from build123d import *

# Parameters (mm, degrees)
SKETCH_1_W                 = 50
SKETCH_1_H                 = 12
UPPER_CROSSBAR_DEPTH       = 28
SKETCH_2_R                 = 9.5
LOWER_GUIDE_SLEEVE_DEPTH   = 5
SKETCH_3_R                 = 6.2
SPINDLE_THROUGH_BORE_DEPTH = 60.774576536
UPPER_HINGE_EAR_DEPTH      = 6.7
SKETCH_6_R                 = 2.6
UPPER_HINGE_BORE_DEPTH     = 59.549124673
EXTRUDE_2_DEPTH            = 6.7
SKETCH_8_R                 = 2.6
CUT_EXTRUDE_2_DEPTH        = 59.549124673
OPPOSITE_HINGE_EAR_DEPTH   = 6.7
SKETCH_10_R                = 2.6
OPPOSITE_HINGE_BORE_DEPTH  = 59.549124673
EXTRUDE_4_DEPTH            = 6.7
SKETCH_12_R                = 2.6
CUT_EXTRUDE_4_DEPTH        = 59.549124673
SKETCH_14_W                = 20
SKETCH_14_H                = 2.2
ARM_SWING_CLEARANCE_DEPTH  = 7.2
SKETCH_15_W                = 20
SKETCH_15_H                = 2.2
CUT_EXTRUDE_6_DEPTH        = 7.2


with BuildPart() as part:
    # 草图1 → Upper_crossbar (new body)
    with BuildSketch(Plane.XY):
        with Locations((25, 6)):
            Rectangle(SKETCH_1_W, SKETCH_1_H)
    extrude(amount=UPPER_CROSSBAR_DEPTH)

    # 草图2 → Lower_guide_sleeve (add)
    with BuildSketch(Plane.XZ):
        with Locations(Location((25, 14, 0), (0, 0, 270))):
            Circle(SKETCH_2_R)
    extrude(amount=LOWER_GUIDE_SLEEVE_DEPTH)

    # 草图3 → Spindle_through_bore (cut, through all)
    with BuildSketch(Plane(origin=(0, 12, 0), x_dir=(1, 0, 0), z_dir=(0, 1, 0))):
        with Locations(Location((25, -14, 0), (0, 0, 270))):
            Circle(SKETCH_3_R)
    extrude(amount=-SPINDLE_THROUGH_BORE_DEPTH, mode=Mode.SUBTRACT)

    # 草图5 → Upper_hinge_ear (add)
    with BuildSketch(Plane.XY.offset(21.3)):
        Polygon((1, -10), (11, -10), (12, -7), (12, 1), (0, 1), (0, -7), align=None)
    extrude(amount=UPPER_HINGE_EAR_DEPTH)

    # 草图6 → Upper_hinge_bore (cut, through all)
    with BuildSketch(Plane.XY.offset(28)):
        with Locations((6, -5)):
            Circle(SKETCH_6_R)
    extrude(amount=-UPPER_HINGE_BORE_DEPTH, mode=Mode.SUBTRACT)

    # 草图7 → 凸台-拉伸2 (add)
    with BuildSketch(Plane.XY.offset(21.3)):
        Polygon((39, -10), (49, -10), (50, -7), (50, 1), (38, 1), (38, -7), align=None)
    extrude(amount=EXTRUDE_2_DEPTH)

    # 草图8 → 切除-拉伸2 (cut, through all)
    with BuildSketch(Plane.XY.offset(28)):
        with Locations((44, -5)):
            Circle(SKETCH_8_R)
    extrude(amount=-CUT_EXTRUDE_2_DEPTH, mode=Mode.SUBTRACT)

    # 草图9 → Opposite_hinge_ear (add)
    with BuildSketch(Plane.XY):
        Polygon((1, -10), (11, -10), (12, -7), (12, 1), (0, 1), (0, -7), align=None)
    extrude(amount=OPPOSITE_HINGE_EAR_DEPTH)

    # 草图10 → Opposite_hinge_bore (cut, through all)
    with BuildSketch(Plane(origin=(0, 0, 0), x_dir=(-1, 0, 0), z_dir=(0, 0, -1))):
        with Locations(Location((-6, -5, 0), (0, 0, 180))):
            Circle(SKETCH_10_R)
    extrude(amount=-OPPOSITE_HINGE_BORE_DEPTH, mode=Mode.SUBTRACT)

    # 草图11 → 凸台-拉伸4 (add)
    with BuildSketch(Plane.XY):
        Polygon((39, -10), (49, -10), (50, -7), (50, 1), (38, 1), (38, -7), align=None)
    extrude(amount=EXTRUDE_4_DEPTH)

    # 草图12 → 切除-拉伸4 (cut, through all)
    with BuildSketch(Plane(origin=(0, 0, 0), x_dir=(-1, 0, 0), z_dir=(0, 0, -1))):
        with Locations(Location((-44, -5, 0), (0, 0, 180))):
            Circle(SKETCH_12_R)
    extrude(amount=-CUT_EXTRUDE_4_DEPTH, mode=Mode.SUBTRACT)

    # 草图14 → Arm_swing_clearance (cut, symmetric)
    with BuildSketch(Plane.XY.offset(14)):
        with Locations((8, 0.9)):
            Rectangle(SKETCH_14_W, SKETCH_14_H)
    extrude(amount=ARM_SWING_CLEARANCE_DEPTH, both=True, mode=Mode.SUBTRACT)

    # 草图15 → 切除-拉伸6 (cut, symmetric)
    with BuildSketch(Plane.XY.offset(14)):
        with Locations((42, 0.9)):
            Rectangle(SKETCH_15_W, SKETCH_15_H)
    extrude(amount=CUT_EXTRUDE_6_DEPTH, both=True, mode=Mode.SUBTRACT)


solid = part.part
Verification items for the finished model (mm, model axes). A direction names the side the tool comes from. Coordinates: 2 decimals unless noted, no trailing zeros. Order: outer loops, then holes, each group sorted by start corner. A loop starts at its lowest first (then second) coordinate and runs counter-clockwise, first axis right, second up.
1. Sectioned sample at B-B, the plane y = -1. Record the cut outline in (x, z).
Results found:
outline: (0, 0) - (12, 0) - (12, 6.7) - (0, 6.7) - close; (0, 21.3) - (12, 21.3) - (12, 28) - (0, 28) - close; circle Ø19 at (25, 14); (38, 0) - (50, 0) - (50, 6.7) - (38, 6.7) - close; (38, 21.3) - (50, 21.3) - (50, 28) - (38, 28) - close; hole circle Ø12.4 at (25, 14)
2. Sectioned sample at C-C, the plane x = 25. Record the cut outline in (y, z).
Results found:
outline: (-5, 4.5) - (0, 4.5) - (0, 0) - (12, 0) - (12, 7.8) - (-5, 7.8) - close; (-5, 20.2) - (12, 20.2) - (12, 28) - (0, 28) - (0, 23.5) - (-5, 23.5) - close
3. Go/stop test with flat-tipped pins: pin 1 Ø1.5 at (y, z) = (-4, 10.5) entering from -X; pin 2 Ø1.5 at (x, z) = (10.5, 16.5) entering from -Y; pin 3 Ø2.5 at (y, z) = (0.5, 13) entering from +X. Record where each tip stops, or that it passes through.
Results found:
pin 1: stops at x = 15.91
pin 2: stops at y = 2
pin 3: stops at x = 34.5
4. Sectioned sample at D-D, the plane z = 24.5. Record the cut outline in (x, y), and give its area (3 significant figures).
Results found:
outline: (0, -7) - (1, -10) - (11, -10) - (12, -7) - (12, 0) - (38, 0) - (38, -7) - (39, -10) - (49, -10) - (50, -7) - (50, 12) - (0, 12) - close; hole circle Ø5.2 at (6, -5); hole circle Ø5.2 at (44, -5)
area: 792 mm2
5. Release check for a two-part mould opening along Z. For faces 1 (the face through (32, 1, 14)), 2 (the face through (25, 4, 0)), 3 (the face through (44, -10, 25)) record: +Z half, -Z half, draft (parallel to the pull), parting line (faces both ways), or undercut.
Results found:
face 1: undercut
face 2: -Z half
face 3: draft
6. Sectioned sample at A-A, the plane z = 14. Record the cut outline in (x, y), and give its area (3 significant figures).
Results found:
outline: (0, 2) - (18, 2) - (18, -0.2) - (15.5, -0.2) - (15.5, -5) - (18.8, -5) - (18.8, 12) - (0, 12) - close; (31.2, -5) - (34.5, -5) - (34.5, -0.2) - (32, -0.2) - (32, 2) - (50, 2) - (50, 12) - (31.2, 12) - close
area: 411 mm2
7. Scan lines: line 1 (X direction, y = -5, z = 4.25); line 2 (Y direction, x = 6, z = 23.5); line 3 (Z direction, x = 47.5, y = -8). Record each from-to range of solid material in increasing order.
Results found:
line 1: x = 0 to 3.4, 8.6 to 12, 38 to 41.4, 46.6 to 50
line 2: y = -10 to -7.6, -2.4 to 12
line 3: z = 0 to 6.7, 21.3 to 28
8. Set-up check for faces 4 (the face through (41, -5, 6.7)), 5 (the face through (9, 1, 6.8)), 6 (the face through (12, -4, 3)): record each of +Z, -Z, +X, -X, +Y, -Y from which the full face is reachable in a straight line by a thin tool's end or side.
Results found:
face 4: +X, -Y
face 5: -X, -Y
face 6: +Z, -Z, -Y
